from build123d import *

# Parameters (mm, degrees)
SKETCH1_W           = 8
SKETCH1_H           = 8
BOSS_EXTRUDE1_DEPTH = 6
SKETCH2_R           = 1.5
CUT_EXTRUDE1_DEPTH  = 6
CUT_EXTRUDE3_DEPTH  = 9
SKETCH4_R           = 1.5
BOSS_EXTRUDE3_DEPTH = 1
FILLET1_R           = 1.5


with BuildPart() as part:
    # Sketch1 → Boss-Extrude1 (new body)
    with BuildSketch(Plane.XY):
        with Locations((4, 4)):
            Rectangle(SKETCH1_W, SKETCH1_H)
    extrude(amount=BOSS_EXTRUDE1_DEPTH)

    # Sketch2 → Cut-Extrude1 (cut)
    with BuildSketch(Plane(origin=(0, 0, 0), x_dir=(-1, 0, 0), z_dir=(0, 0, -1))):
        with Locations((-5.5, 4)):
            Circle(SKETCH2_R)
    extrude(amount=-CUT_EXTRUDE1_DEPTH, mode=Mode.SUBTRACT)

    # Sketch3 → Cut-Extrude3 (cut)
    with BuildSketch(Plane.XZ):
        with BuildLine():
            Line((0, 6), (0, 0))
            ThreePointArc((0, 0), (3, 3), (0, 6))
        make_face()
    extrude(amount=-CUT_EXTRUDE3_DEPTH, mode=Mode.SUBTRACT)

    # Sketch4 → Boss-Extrude3 (add)
    with BuildSketch(Plane(origin=(0, 0, 0), x_dir=(-1, 0, 0), z_dir=(0, 0, -1))):
        with Locations((-5.5, 4)):
            Circle(SKETCH4_R)
    extrude(amount=-BOSS_EXTRUDE3_DEPTH)

    # Fillet1
    fillet1_edges = [part.edges().sort_by_distance(p)[0] for p in [
        (8, 8, 3),
        (8, 0, 3),
    ]]
    fillet(fillet1_edges, radius=FILLET1_R)


solid = part.part
Input: part model. Units: mm. Frame: model coordinates. A direction names the side the tool comes from. Round coordinates to 2 decimals unless told otherwise and drop trailing zeros. Write each loop counter-clockwise with the first axis right and the second up, starting at its lowest first coordinate (ties: lowest second). Pieces come first, ordered by that corner, then holes.
1) Contact query for flat-ended pins moving along their axis: P1, Ø2.5, axis at x = 5.5, y = 4, coming from the +Z side; P2, Ø2.5, axis at x = 6, y = 3.5, coming from the +Z side. Output: stop coordinate, or through.
2) Ray query, L1, parallel to Y at x = 5.5, z = 2.7; L2, parallel to Z at x = 5.25, y = 3.5; L3, parallel to X at y = 3.5, z = 5.5. Return the intervals inside material, ascending.
3) Cut plane A-A (z = 1.2). Return the cut outline in (x, y).
4) Cut plane C-C (y = 4). Return the cut outline in (x, z), then the cut area to 3 significant figures.
5) Reachability of faces 1 (the flat face through (3, 4, 6)), 2 (the cylindrical face through (6.61, 5.01, 3.46)) from +Z, -Z, +X, -X, +Y, -Y: full face, straight path, thin tool, end or side. Return the list, or none.
6) Draft query along X for faces 3 (the flat face through (6, 4, 1)), 4 (the cylindrical face through (7.55, 0.43, 3.04)), 5 (the flat face through (5, 8, 3)). Return one class per face: pulls with the +X half, pulls with the -X half, needs draft (parallel to the pull), parting line crosses it, or undercut.
7) Cut plane D-D (x = 1). Return the cut outline in (y, z).
8) Cut plane B-B (x = 5.5). Return the cut outline in (y, z), then the cut area to 3 significant figures.
Geometry says:
1. P1: stops at z = 1
1. P2: stops at z = 6
2. L1: y = 0 to 2.5, 5.5 to 8
2. L2: z = 0 to 1
2. L3: x = 1.66 to 4.09, 6.91 to 8
3. outline: (2.4, 0) - (6.5, 0) arc R1.5 ccw to (8, 1.5) - (8, 6.5) arc R1.5 ccw to (6.5, 8) - (2.4, 8) - close; hole circle Ø3 at (5.5, 4)
4. outline: (0, 0) - (8, 0) - (8, 6) - (7, 6) - (7, 1) - (4, 1) - (4, 6) - (0, 6) arc R3 cw to start
4. area: 18.9 mm2
5. face 1: +Z, +X, -X, +Y, -Y
5. face 2: +Z
6. face 3: undercut
6. face 4: pulls with the +X half
6. face 5: needs draft
7. outline: (0, 0) - (8, 0) - (8, 0.17) - (0, 0.17) - close; (0, 5.83) - (8, 5.83) - (8, 6) - (0, 6) - close
8. outline: (0, 0) - (8, 0) - (8, 6) - (5.5, 6) - (5.5, 1) - (2.5, 1) - (2.5, 6) - (0, 6) - close
8. area: 33.0 mm2
